```python
from build123d import *

# Parameters (mm, degrees)
F0_W     = 98.002754
F0_H     = 56.256722
F1_DEPTH = 25.4
F2_T     = -2.54
F3_W     = 11.132365
F3_H     = 18.58267
F4_DEPTH = 27.40012


with BuildPart() as f1:
    # F0 (on Front) → F1 (new body)
    with BuildSketch(Plane.XZ):
        Rectangle(F0_W, F0_H)
    extrude(amount=F1_DEPTH)

    # F2
    f2_openings = [f1.faces().sort_by_distance(p)[0] for p in [
        (0, -25.4, 0),
    ]]
    offset(amount=F2_T, openings=f2_openings)

    # F3 (on face) → F4 (join)
    with BuildSketch(Plane.YZ.offset(-46.461377)):
        with Locations((-14.144399, 5.063872)):
            Rectangle(F3_W, F3_H)
    extrude(amount=-F4_DEPTH)


solid = f1.part
```
Check sheet for the modelled part. Datum: model origin and axes. Units: mm. A direction names the side the tool comes from. Coordinates: 2 decimals unless noted, no trailing zeros. Loops run counter-clockwise (first coordinate to the right, second up) from the corner with the lowest first, then second, coordinate; pieces in that order, holes last. Notation, with made-up numbers: M 83,-6 L 137,-6 A18 ccw 137,0 Z; hole C -7.75,29.25 d4. An arc over 180 degrees is marked long. Answer as a JSON object with one key per item and string values.
1. Sectioned sample at C-C on z = -20. Record the cut outline in (x, y).
Outcome:
{"outline": "M -49,-25.4 L -46.46,-25.4 L -46.46,-2.54 L 46.46,-2.54 L 46.46,-25.4 L 49,-25.4 L 49,0 L -49,0 Z"}
2. Sectioned sample at D-D on y = -4.75. Record the cut outline in (x, z), and give its area (3 significant figures).
Outcome:
{"outline": "M -49,-28.13 L 49,-28.13 L 49,28.13 L -49,28.13 Z; hole M -46.46,-25.59 L 46.46,-25.59 L 46.46,25.59 L -46.46,25.59 Z", "area": "758 mm²"}
3. Depth check by flat-ended pin: P1, Ø12, axis at x = 3.5, z = 14, coming from the -Y side; P2, Ø12.5, axis at y = -14.5, z = -11.5, coming from the -X side; P3, Ø5.5, axis at x = -56.5, y = -11.5, coming from the +Z side. Enter the tip coordinate at first touch or a pass-through.
Outcome:
{"P1": "y = -2.54", "P2": "x = -49", "P3": "z = 14.36"}
4. Release check for a two-part mould opening along X. For faces 1 (the flat face through (49.001, -13, 0)), 2 (the flat face through (-1, -14, -25.588)), 3 (the flat face through (-1, -13, 28.128)) record: pulls with the +X half, pulls with the -X half, needs draft (parallel to the pull), parting line crosses it, or undercut.
Outcome:
{"face 1": "pulls with the +X half", "face 2": "undercut", "face 3": "needs draft"}
5. Sectioned sample at B-B on x = -35.5. Record the cut outline in (y, z).
Outcome:
{"outline": "M -25.4,-28.13 L 0,-28.13 L 0,28.13 L -25.4,28.13 L -25.4,25.59 L -2.54,25.59 L -2.54,-25.59 L -25.4,-25.59 Z"}
6. Sectioned sample at A-A on y = -16. Record the cut outline in (x, z).
Outcome:
{"outline": "M -73.86,-4.23 L -49,-4.23 L -49,-28.13 L 49,-28.13 L 49,28.13 L -49,28.13 L -49,14.36 L -73.86,14.36 Z; hole M -46.46,-25.59 L 46.46,-25.59 L 46.46,25.59 L -46.46,25.59 Z"}
7. Scan lines: L1, parallel to Z at x = -31, y = -8.5; L2, parallel to X at y = -24, z = -16.5; L3, parallel to X at y = -13.5, z = 0. Record each from-to range of solid material in increasing order. Write a range as from..to.
Outcome:
{"L1": "-28.13..-25.59, 25.59..28.13", "L2": "-49..-46.46, 46.46..49", "L3": "-73.86..-46.46, 46.46..49"}
8. Access from +Z, -Z, +X, -X, +Y, -Y to the whole of each face (thin tool, end or side, straight path). Record for faces 4 (the flat face through (-61, -14, -4.227)), 5 (the flat face through (-61, -19.711, 5)), 6 (the flat face through (46.461, -14, 0)).
Outcome:
{"face 4": "-Z, -X, +Y, -Y", "face 5": "+Z, -Z, -X, -Y", "face 6": "-Y"}
